The model under review builds one solid part; all positions refer to its coordinate system, in mm. Give positions to 0.01 mm unless a question says otherwise; leave off trailing zeros. Loops run counter-clockwise (first coordinate to the right, second up) from the corner with the lowest first, then second, coordinate; pieces in that order, holes last. Notation, with made-up numbers: (15.5, 0) - (19.5, 0) arc R19 ccw to (19.5, 31) - close; hole circle Ø2 at (49.25, 82). An arc over 180 degrees is marked (long way). Answer as a JSON object with one key per item and string values.
from build123d import *

# Parameters (mm, degrees)
SKETCH1_R           = 13
SKETCH1_R_2         = 10
BOSS_EXTRUDE1_DEPTH = 700
CUT_EXTRUDE1_START  = -20
CUT_EXTRUDE1_DEPTH  = 20
CUT_EXTRUDE2_DEPTH  = 20


with BuildPart() as part:
    # Sketch1 → Boss-Extrude1 (new body)
    with BuildSketch(Plane.XY):
        Circle(SKETCH1_R)
        Circle(SKETCH1_R_2, mode=Mode.SUBTRACT)
    extrude(amount=BOSS_EXTRUDE1_DEPTH)

    # Sketch2 → Cut-Extrude1 (cut)
    with BuildSketch(Plane.XY.offset(700).offset(CUT_EXTRUDE1_START)):
        with BuildLine():
            Line((-1, 9.949874371), (-1, 12))
            Line((-1, 12), (1, 12))
            Line((1, 12), (1, 9.949874371))
            ThreePointArc((1, 9.949874371), (0, 10), (-1, 9.949874371))
        make_face()
    extrude(amount=CUT_EXTRUDE1_DEPTH, mode=Mode.SUBTRACT)

    # Sketch3 → Cut-Extrude2 (cut)
    with BuildSketch(Plane(origin=(0, 0, 0), x_dir=(-1, 0, 0), z_dir=(0, 0, -1))):
        with BuildLine():
            Line((-1, 9.949874371), (-1, 11.949874371))
            Line((-1, 11.949874371), (1, 11.949874371))
            Line((1, 11.949874371), (1, 9.949874371))
            ThreePointArc((1, 9.949874371), (0, 10), (-1, 9.949874371))
        make_face()
    extrude(amount=-CUT_EXTRUDE2_DEPTH, mode=Mode.SUBTRACT)


solid = part.part
Q1. Clearance check with flat-ended pins moving along their axes: pin 1 Ø1.6 at (y, z) = (10.5, 688.5) entering from -X; pin 2 Ø1 at (y, z) = (2.5, 308.5) entering from +X; pin 3 Ø6 at (x, z) = (5, 434) entering from -Y. State where each tip first meets the part, or that it passes through.
Results:
{"pin 1": "stops at x = -8.66", "pin 2": "stops at x = 12.85", "pin 3": "stops at y = -12.85"}
Q2. To check wall thickness, follow probe 1 along Y at (x, z) = (0, 417); probe 2 along X at (y, z) = (0.75, 60); probe 3 along X at (y, z) = (6.5, 256.5). State the ranges of each line that lie inside material, in increasing order. Write a range as [from, to].
Results:
{"probe 1": "y = [-13, -10], [10, 13]", "probe 2": "x = [-12.98, -9.97], [9.97, 12.98]", "probe 3": "x = [-11.26, -7.6], [7.6, 11.26]"}
Q3. The part is to be moulded in two halves that separate along X. For faces 1 (the face through (10, 3, 700)), 2 (the face through (-10.316, -7.91, 345.1)), 3 (the face through (-2.17, -9.76, 345.1)), say which applies: +X half, -X half, draft (parallel to the pull), parting line (faces both ways), or undercut.
Results:
{"face 1": "draft", "face 2": "parting line", "face 3": "undercut"}
Q4. Consider section A-A, the plane y = 0. State the section outline as (x, z) points.
Results:
{"outline": "(-13, 0) - (-10, 0) - (-10, 700) - (-13, 700) - close; (10, 0) - (13, 0) - (13, 700) - (10, 700) - close"}
Q5. Consider section B-B, the plane z = 123.5. State the section outline as (x, y) points, plus the area to 3 significant figures.
Results:
{"outline": "circle Ø26 at (0, 0); hole circle Ø20 at (0, 0)", "area": "217 mm^2"}
